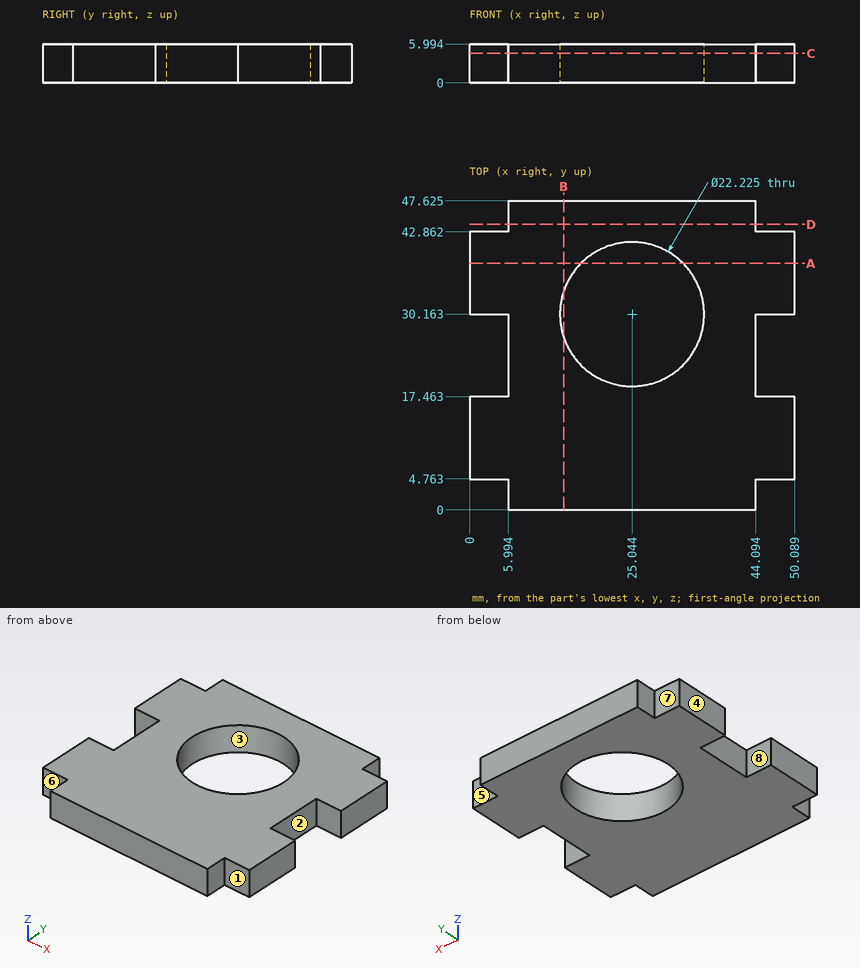
Source: three-view drawing plus pictorial views. Frame: mm from the lowest corner of the part. A direction names the side the tool comes from. Give positions to 0.01 mm unless a question says otherwise; leave off trailing zeros. Loops run counter-clockwise (first coordinate to the right, second up) from the corner with the lowest first, then second, coordinate; pieces in that order, holes last. Notation, with made-up numbers: M -6.5,-12.5 L 15.5,-12.5 A29 cw 15.5,10.5 Z; hole C 49,-27.5 d11. An arc over 180 degrees is marked long. Put each result on its own line as item: value.
Q1. Section B-B (x = 14.5). Return the cut outline in (y, z) (1 decimal).
Response values:
outline: M 0,0 L 26.7,0 L 26.7,6 L 0,6 Z; M 33.7,0 L 47.6,0 L 47.6,6 L 33.7,6 Z
Q2. Line query: probe 1 along Y at (x, z) = (45, 1); probe 2 along X at (y, z) = (30, 4.25) (1 decimal); probe 3 along Y at (x, z) = (17.5, 0.65) (1 decimal). Output: solid intervals per line, ascending. Write a range as [from, to].
Response values:
probe 1: y = [4.76, 17.46], [30.16, 42.86]
probe 2: x = [6, 13.9], [36.2, 44.1]
probe 3: y = [0, 22], [38.3, 47.6]
Q3. Section D-D (y = 44). Return the cut outline in (x, z) (1 decimal).
Response values:
outline: M 6,0 L 44.1,0 L 44.1,6 L 6,6 Z
Q4. Section C-C (z = 4.55). Return the cut outline in (x, y) (1 decimal), and give its area (3 significant figures).
Response values:
outline: M 0,4.8 L 6,4.8 L 6,0 L 44.1,0 L 44.1,4.8 L 50.1,4.8 L 50.1,17.5 L 44.1,17.5 L 44.1,30.2 L 50.1,30.2 L 50.1,42.9 L 44.1,42.9 L 44.1,47.6 L 6,47.6 L 6,42.9 L 0,42.9 L 0,30.2 L 6,30.2 L 6,17.5 L 0,17.5 Z; hole C 25,30.2 d22.2
area: 1,730 mm²
Q5. Section A-A (y = 38). Return the cut outline in (x, z) (1 decimal).
Response values:
outline: M 0,0 L 17.2,0 L 17.2,6 L 0,6 Z; M 32.9,0 L 50.1,0 L 50.1,6 L 32.9,6 Z
Q6. Pin query (flat end, axial travel): P1, Ø3, axis at x = 48, z = 2.5, coming from the -Y side; P2, Ø1.8, axis at x = 47.5, z = 4, coming from the +Y side; P3, Ø1.4, axis at y = 45, z = 3, coming from the -X side. Return the tip coordinate at first contact, or that it passes through.
Response values:
P1: stops at y = 4.76
P2: stops at y = 42.86
P3: stops at x = 5.99
Q7. Mould query, pull axis Y, two halves, no side actions, for the marked faces 1, 2, 3 and 4. Classes: released by +Y, released by -Y, zero draft, split by the parting line, or undercut.
Response values:
face 1: released by -Y
face 2: undercut
face 3: undercut
face 4: zero draft
Q8. Reachability of the marked faces 5, 6, 7 and 8 from +Z, -Z, +X, -X, +Y, -Y: full face, straight path, thin tool, end or side. Return the list, or none.
Response values:
face 5: +Z, -Z, +X, +Y
face 6: +Z, -Z, -X, -Y
face 7: +Z, -Z, -X, +Y
face 8: +Z, -Z, -X
